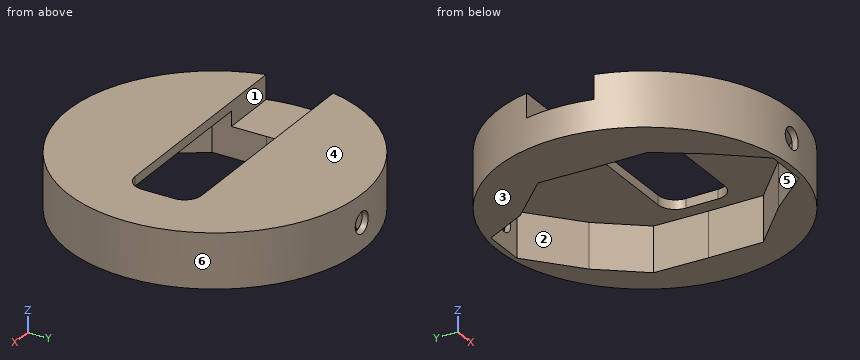
```python
from build123d import *

# Parameters (mm, degrees)
F0_R          = 68.5
F1_DEPTH      = 25.4
F3_DEPTH      = 11.25
F6_DEPTH      = 21.082
F4_R          = 5
F7_DEPTH      = 68.501
F7_DEPTH_BACK = 68.501


with BuildPart() as f1:
    # F0 (on Top) → F1 (new body)
    with BuildSketch(Plane.XY):
        Circle(F0_R)
    extrude(amount=F1_DEPTH)

    # F2 (on face) → F3 (cut)
    with BuildSketch(Plane.XY.offset(25.4)):
        with BuildLine():
            Line((34.15, 14.5270901566), (-88.2992463768, 14.5270901566))
            Line((-88.2992463768, 14.5270901566), (-88.2992463768, -16.4609098434))
            Line((-88.2992463768, -16.4609098434), (34.15, -16.4609098434))
            ThreePointArc((34.15, -16.4609098434), (39.8068542495, -14.1177640929), (42.15, -8.4609098434))
            Line((42.15, -8.4609098434), (42.15, 6.5270901566))
            ThreePointArc((42.15, 6.5270901566), (39.8068542495, 12.183944406), (34.15, 14.5270901566))
        make_face()
    extrude(amount=-F3_DEPTH, mode=Mode.SUBTRACT)

    # F5 (on face) → F6 (cut)
    with BuildSketch(Plane(origin=(0, 0, 0), x_dir=(1, 0, 0), z_dir=(0, 0, -1))):
        Polygon((10.1280519739, 65.532), (-9.8341628909, 65.532), (-25.9055476636, 45.72), (-39.7767797112, 25.4), (-39.7767797112, 0), (-40.3115227818, -25.4), (-20.4457305372, -45.72), (-10.3001166135, -65.532), (9.6642833865, -65.532), (32.5386694628, -45.72), (48.4360772182, -25.4), (48.9794053137, 0), (48.9794053137, 25.4), (27.0890761167, 45.72), align=None)
    extrude(amount=-F6_DEPTH, mode=Mode.SUBTRACT)

    # F4 (on Front) → F7 (cut, two sides)
    with BuildSketch(Plane.XZ) as f7_sk:
        with Locations((0, 12.5027870712)):
            Circle(F4_R)
    extrude(amount=-F7_DEPTH, mode=Mode.SUBTRACT)
    extrude(f7_sk.sketch, amount=F7_DEPTH_BACK, mode=Mode.SUBTRACT)


solid = f1.part
```
CAD build for the part. Positions are in the model's coordinates, mm. Face numbers are marked on the shaded views. A direction names the side the tool comes from. Round coordinates to 2 decimals unless told otherwise and drop trailing zeros. Write each loop counter-clockwise with the first axis right and the second up, starting at its lowest first coordinate (ties: lowest second). Pieces come first, ordered by that corner, then holes. Notation, with made-up numbers: (53.5, 80.25) -> (78.5, 80.25) arc R22 ccw to (78.5, 117.25) -> close; hole circle Ø3 at (-22, -15). An arc over 180 degrees is marked (long way). Answer in a Markdown table with one row per item. Add a question column.
Item 1: Saw through at A-A, the plane x = 0. Write the cut outline in (y, z), then the cut area to 3 significant figures.
Item 2: Saw through at B-B, the plane z = 4.75. Write the cut outline in (x, y).
Item 3: Drill centre lines: line 1 (Z direction, x = 0, y = -66); line 2 (X direction, y = -0.5, z = 5.5); line 3 (Z direction, x = 1, y = 61). Where is each one in solid material? Low to high. Write a range as from..to.
Item 4: Mould opens along X. For the marked faces 4, 5 and 6 say: pulls with the +X half, pulls with the -X half, needs draft (parallel to the pull), parting line crosses it, or undercut.
Item 5: Which spindle directions (+Z, -Z, +X, -X, +Y, -Y) get a long thin tool onto all of the face, cutting with end or side? Do the marked faces 1, 2 and 3. Say none if no direction does.
Item 6: Saw through at C-C, the plane y = -52.5. Write the cut outline in (x, z), then the cut area to 3 significant figures.
Item 7: Drop flat-ended pins along their axis: pin 1 Ø10 at (y, z) = (54.5, 7.5) entering from -X; pin 2 Ø5.5 at (x, z) = (-14.5, 18) entering from -Y; pin 3 Ø3.5 at (x, z) = (-39, 17) entering from +Y; pin 4 Ø8 at (x, z) = (0, 12.5) entering from -Y. Give the stop position or say it passes through.
Item 8: Saw through at D-D, the plane x = 23.5. Write the cut outline in (y, z).
Findings below:
| question | item | result |
|---|---|---|
| 1 | outline | (-68.5, 0) -> (-65.53, 0) -> (-65.53, 7.5) -> (-68.5, 7.5) -> close; (-68.5, 17.5) -> (-65.53, 17.5) -> (-65.53, 21.08) -> (-16.46, 21.08) -> (-16.46, 25.4) -> (-68.5, 25.4) -> close; (14.53, 21.08) -> (65.53, 21.08) -> (65.53, 17.5) -> (68.5, 17.5) -> (68.5, 25.4) -> (14.53, 25.4) -> close; (65.53, 0) -> (68.5, 0) -> (68.5, 7.5) -> (65.53, 7.5) -> close |
| 1 | area | 524 mm^2 |
| 2 | outline | circle Ø137 at (0, 0); hole (-40.31, 25.4) -> (-39.78, 0) -> (-39.78, -25.4) -> (-25.91, -45.72) -> (-9.83, -65.53) -> (10.13, -65.53) -> (27.09, -45.72) -> (48.98, -25.4) -> (48.98, 0) -> (48.44, 25.4) -> (32.54, 45.72) -> (9.66, 65.53) -> (-10.3, 65.53) -> (-20.45, 45.72) -> close |
| 3 | line 1 | z = 0..7.5, 17.5..25.4 |
| 3 | line 2 | x = -68.5..-39.78, 48.98..68.5 |
| 3 | line 3 | z = 21.08..25.4 |
| 4 | face 4 | needs draft |
| 4 | face 5 | undercut |
| 4 | face 6 | parting line crosses it |
| 5 | face 1 | +Z, -X |
| 5 | face 2 | -Z |
| 5 | face 3 | -Z, +X, -X, +Y, -Y |
| 6 | outline | (-44, 0) -> (-20.41, 0) -> (-20.41, 21.08) -> (21.28, 21.08) -> (21.28, 0) -> (44, 0) -> (44, 25.4) -> (-44, 25.4) -> close |
| 6 | area | 1,360 mm^2 |
| 7 | pin 1 | stops at x = -47.35 |
| 7 | pin 2 | stops at y = -67.48 |
| 7 | pin 3 | stops at y = 57.49 |
| 7 | pin 4 | passes through |
| 8 | outline | (-64.34, 0) -> (-49.91, 0) -> (-49.91, 21.08) -> (-16.46, 21.08) -> (-16.46, 25.4) -> (-64.34, 25.4) -> close; (14.53, 21.08) -> (53.55, 21.08) -> (53.55, 0) -> (64.34, 0) -> (64.34, 25.4) -> (14.53, 25.4) -> close |
